from build123d import *

# Parameters (mm, degrees)
F0_R     = 11.5
F0_R_2   = 0.5
F0_R_3   = 1.05
F0_W     = 5
F0_H     = 5
F1_DEPTH = 0.8
F2_DEPTH = 1.2


with BuildPart() as f1:
    # F0 (on Top) → F1 (new body)
    with BuildSketch(Plane.XY):
        Circle(F0_R)
        Polygon((-4.980064, -3.625723), (-0.649936, -6.125723), (-3.149936, -10.45585), (-7.480064, -7.95585), align=None, mode=Mode.SUBTRACT)
        with Locations((-0.092426, -4.110796)):
            Circle(F0_R_2, mode=Mode.SUBTRACT)
        with Locations((-4.127668, -1.922055)):
            Circle(F0_R_2, mode=Mode.SUBTRACT)
        with Locations((0.046018, -9.505966)):
            Circle(F0_R_3, mode=Mode.SUBTRACT)
        Polygon((0.649936, -6.125723), (4.980064, -3.625723), (7.480064, -7.95585), (3.149936, -10.45585), align=None, mode=Mode.SUBTRACT)
        with Locations((4.24384, -2.238264)):
            Circle(F0_R_2, mode=Mode.SUBTRACT)
        with Locations((-8.13, 0)):
            Rectangle(F0_W, F0_H, mode=Mode.SUBTRACT)
        with Locations((-3.94603, 2.246665)):
            Circle(F0_R_2, mode=Mode.SUBTRACT)
        Polygon((-0.649936, 6.125723), (-4.980064, 3.625723), (-7.480064, 7.95585), (-3.149936, 10.45585), align=None, mode=Mode.SUBTRACT)
        Rectangle(F0_W, F0_H, mode=Mode.SUBTRACT)
        with Locations((4.07016, 2.455426)):
            Circle(F0_R_2, mode=Mode.SUBTRACT)
        with Locations((8.13, 0)):
            Rectangle(F0_W, F0_H, mode=Mode.SUBTRACT)
        Polygon((4.980064, 3.625723), (0.649936, 6.125723), (3.149936, 10.45585), (7.480064, 7.95585), align=None, mode=Mode.SUBTRACT)
        with Locations((0.057833, 9.808174)):
            Circle(F0_R_3, mode=Mode.SUBTRACT)
        Polygon((-7.480064, 7.95585), (-4.980064, 3.625723), (-0.649936, 6.125723), (-3.149936, 10.45585), align=None)
        Polygon((3.149936, 10.45585), (0.649936, 6.125723), (4.980064, 3.625723), (7.480064, 7.95585), align=None)
        with Locations((8.13, 0)):
            Rectangle(F0_W, F0_H)
        with Locations((-8.13, 0)):
            Rectangle(F0_W, F0_H)
        Rectangle(F0_W, F0_H)
        Polygon((-3.149936, -10.45585), (-0.649936, -6.125723), (-4.980064, -3.625723), (-7.480064, -7.95585), align=None)
        Polygon((7.480064, -7.95585), (4.980064, -3.625723), (0.649936, -6.125723), (3.149936, -10.45585), align=None)
    extrude(amount=-F1_DEPTH)

    # F0 (on Top) → F2 (join)
    with BuildSketch(Plane.XY):
        Polygon((-7.480064, 7.95585), (-4.980064, 3.625723), (-0.649936, 6.125723), (-3.149936, 10.45585), align=None)
        Polygon((3.149936, 10.45585), (0.649936, 6.125723), (4.980064, 3.625723), (7.480064, 7.95585), align=None)
        with Locations((-8.13, 0)):
            Rectangle(F0_W, F0_H)
        Rectangle(F0_W, F0_H)
        with Locations((8.13, 0)):
            Rectangle(F0_W, F0_H)
        Polygon((-3.149936, -10.45585), (-0.649936, -6.125723), (-4.980064, -3.625723), (-7.480064, -7.95585), align=None)
        Polygon((7.480064, -7.95585), (4.980064, -3.625723), (0.649936, -6.125723), (3.149936, -10.45585), align=None)
    extrude(amount=F2_DEPTH)


solid = f1.part
For this review, take the finished solid that the model builds, in its own axes (mm). A direction names the side the tool comes from. Give positions to 0.01 mm unless a question says otherwise; leave off trailing zeros. Loops run counter-clockwise (first coordinate to the right, second up) from the corner with the lowest first, then second, coordinate; pieces in that order, holes last. Notation, with made-up numbers: M -11.5,49 L -4.5,49 A7 ccw -4.5,56 Z; hole C 52.5,0.25 d10. An arc over 180 degrees is marked long. Answer as a JSON object with one key per item and string values. Group by question number.
Q1. Add section A-A on z = 0.7. Give the boundary of the cut face in (x, y).
Q2. Add section B-B on y = 0. Give the boundary of the cut face in (x, z).
Q3. Mouldability with a two-part tool opening along X and no side actions: class faces 4 (the cylindrical face through (-1.5, 11.4, -0.4)), 5 (the flat face through (5.345, 9.188, 0.592)), 6 (the cylindrical face through (-3.65, -1.77, -0.39)), 7 (the flat face through (8, 2.5, 1)) as +X half, -X half, draft (parallel to the pull), parting line (faces both ways), or undercut.
Q4. Insertion check: P1, Ø1, axis at y = 0.5, z = 1, coming from the +X side; P2, Ø0.6, axis at x = -8, z = 1, coming from the -Y side; P3, Ø3.5, axis at x = 0.06, y = 9.81, coming from the +Z side. Each pin has a flat end and moves straight along its axis. Give the tip position at first contact, or say it passes through.
Q5. Tool access review of faces 1 (the flat face through (0, 2.5, 1)), 2 (the flat face through (-5.63, 0, 1)), 3 (the flat face through (10.63, 0, 1)): name each direction out of +Z, -Z, +X, -X, +Y, -Y from which nothing blocks a thin tool from reaching the whole face with its end or side.
Q6. Add section C-C on x = 0. Give the boundary of the cut face in (y, z), and give its area (3 significant figures).
Q7. For probe 1 along X at (y, z) = (2.5, -0.3); probe 2 along Y at (x, z) = (-6.5, 0.7); probe 3 along Y at (x, z) = (-1.25, 0.9), list the stretches that pass through material, from the lowest coordinate up. Write a range as [from, to].
Q8. Add section D-D on y = -10. Give the boundary of the cut face in (x, z), and give its area (3 significant figures).
Checked values:
{
 "1": {"outline": "M -10.63,-2.5 L -5.63,-2.5 L -5.63,2.5 L -10.63,2.5 Z; M -7.48,-7.96 L -3.15,-10.46 L -0.65,-6.13 L -4.98,-3.63 Z; M -7.48,7.96 L -4.98,3.63 L -0.65,6.13 L -3.15,10.46 Z; M -2.5,-2.5 L 2.5,-2.5 L 2.5,2.5 L -2.5,2.5 Z; M 0.65,-6.13 L 3.15,-10.46 L 7.48,-7.96 L 4.98,-3.63 Z; M 0.65,6.13 L 4.98,3.63 L 7.48,7.96 L 3.15,10.46 Z; M 5.63,-2.5 L 10.63,-2.5 L 10.63,2.5 L 5.63,2.5 Z"},
 "2": {"outline": "M -11.5,-0.8 L 11.5,-0.8 L 11.5,0 L 10.63,0 L 10.63,1.2 L 5.63,1.2 L 5.63,0 L 2.5,0 L 2.5,1.2 L -2.5,1.2 L -2.5,0 L -5.63,0 L -5.63,1.2 L -10.63,1.2 L -10.63,0 L -11.5,0 Z"},
 "3": {"face 4": "parting line", "face 5": "+X half", "face 6": "undercut", "face 7": "draft"},
 "4": {"P1": "x = 10.63", "P2": "y = -2.5", "P3": "z = 0"},
 "5": {"face 1": "+Z, +X, -X", "face 2": "+Z", "face 3": "+Z, +X, +Y, -Y"},
 "6": {"outline": "M -11.5,-0.8 L -10.55,-0.8 L -10.55,0 L -11.5,0 Z; M -8.46,-0.8 L -4.6,-0.8 L -4.6,0 L -8.46,0 Z; M -3.62,-0.8 L 8.76,-0.8 L 8.76,0 L 2.5,0 L 2.5,1.2 L -2.5,1.2 L -2.5,0 L -3.62,0 Z; M 10.86,-0.8 L 11.5,-0.8 L 11.5,0 L 10.86,0 Z", "area": "20.3 mm²"},
 "7": {"probe 1": "[-11.22, -4.38], [-3.51, 3.57], [4.57, 11.22]", "probe 2": "[-8.52, -6.26], [-2.5, 2.5], [6.26, 8.52]", "probe 3": "[-7.17, -5.78], [-2.5, 2.5], [5.78, 7.17]"},
 "8": {"outline": "M -5.68,-0.8 L -0.88,-0.8 L -0.88,0 L -2.89,0 L -2.89,1.2 L -3.94,1.2 L -3.94,0 L -5.68,0 Z; M 0.97,-0.8 L 5.68,-0.8 L 5.68,0 L 3.94,0 L 3.94,1.2 L 2.89,1.2 L 2.89,0 L 0.97,0 Z", "area": "10.1 mm²"}
}
